from build123d import *

# Parameters (mm, degrees)
SKETCH1_R           = 23
BOSS_EXTRUDE1_DEPTH = 12
CUT_EXTRUDE1_DEPTH  = 13


with BuildPart() as part:
    # Sketch1 → Boss-Extrude1 (new body)
    with BuildSketch(Plane.XY):
        Circle(SKETCH1_R)
    extrude(amount=BOSS_EXTRUDE1_DEPTH)

    # Sketch2 → Cut-Extrude1 (cut, through all)
    with BuildSketch(Plane.XY.offset(12)):
        with BuildLine():
            Line((-1.669663439, 1.682), (1.669663439, 1.682))
            ThreePointArc((1.669663439, 1.682), (2.259858272, -0.714101248), (0.4, -2.336000856))
            Line((0.4, -2.336000856), (0.4, -5))
            Line((0.4, -5), (6.939400576, -5))
            add(Edge.make_bspline(
                [(-6.939400576, -5), (-6.939400576, -23.218031299), (0, -23.218031299), (6.939400576, -23.218031299), (6.939400576, -5)],
                knots=[1.570796327, 1.570796327, 1.570796327, 3.141592654, 3.141592654, 4.71238898, 4.71238898, 4.71238898], degree=2, weights=[1, 0.707106781, 1, 0.707106781, 1]))
            Line((-6.939400576, -5), (-0.4, -5))
            Line((-0.4, -5), (-0.4, -2.336000856))
            ThreePointArc((-0.4, -2.336000856), (-2.259858272, -0.714101248), (-1.669663439, 1.682))
        make_face()
        with BuildLine():
            Line((-6.939400576, 5), (6.939400576, 5))
            add(Edge.make_bspline(
                [(6.939400576, 5), (5.785687162, 25.074195607), (0, 25.074195607), (-5.785687162, 25.074195607), (-6.939400576, 5)],
                knots=[4.913142926, 4.913142926, 4.913142926, 6.283185307, 6.283185307, 7.653227688, 7.653227688, 7.653227688], degree=2, weights=[1, 0.77440564, 1, 0.77440564, 1]))
        make_face()
    extrude(amount=-CUT_EXTRUDE1_DEPTH, mode=Mode.SUBTRACT)


solid = part.part
Model file for the job. Use its own axes, mm. A direction names the side the tool comes from. Give positions to 0.01 mm unless a question says otherwise; leave off trailing zeros. Order: outer loops, then holes, each group sorted by start corner. A loop starts at its lowest first (then second) coordinate and runs counter-clockwise, first axis right, second up. Notation, with made-up numbers: M -36,-17 L -13,-17 A34 cw -13,17 Z; hole C -36.75,-12 d5. An arc over 180 degrees is marked long. Put each result on its own line as item: value. Start each with the question number.
(1) Tool access for faces 1 (the face through (22.96, -1.38, 5.92)), 2 (the face through (0, 1.682, 6)), 3 (the face through (0.4, -4, 6)): list every direction of +Z, -Z, +X, -X, +Y, -Y with a clear straight run to the whole face (end or side of a thin tool).
(2) Drill centre lines: L1, parallel to X at y = 0, z = 1.25; L2, parallel to X at y = -17.5, z = 7.75; L3, parallel to Y at x = 17, z = 0.5. Where is each one in solid material? Low to high. Write a range as [from, to].
(3) Pin check, flat tips, straight feed: pin 1 Ø1 at (x, z) = (-0.5, 6.5) entering from -Y; pin 2 Ø2 at (x, z) = (3.5, 5.5) entering from -Y; pin 3 Ø1 at (x, z) = (-11.5, 3) entering from +Y; pin 4 Ø6 at (x, z) = (2.5, 4.5) entering from +Y. Stop position of each tip, or through.
(4) Band-saw the part on D-D on x = -12.5. Give the cut face in (y, z).
(5) Band-saw the part on A-A on x = -6. Count the separate pieces of the cut face and the enclosed holes in it, then the cut area to 3 significant figures.
(6) Band-saw the part on B-B on x = 9. Give the cut face in (y, z).
(7) Pull direction Y, two halves, no side cores. Call faces 4 (the face through (-2.25, -0.75, 6.08)), 5 (the face through (-23, 0, 6)), 6 (the face through (5, 0, 12)), 7 (the face through (4, -5, 6)): released by +Y, released by -Y, zero draft, split by the parting line, or undercut.
Results below:
1. face 1: +Z, -Z, +X
1. face 2: +Z, -Z
1. face 3: +Z, -Z, -Y
2. L1: x = [-23, -2.37], [2.37, 23]
2. L2: x = [-14.92, -5.05], [5.05, 14.92]
2. L3: y = [-15.49, 15.49]
3. pin 1: stops at y = -5
3. pin 2: stops at y = -22.86
3. pin 3: stops at y = 20.2
3. pin 4: stops at y = 22.81
4. outline: M -19.31,0 L 19.31,0 L 19.31,12 L -19.31,12 Z
5. separate pieces: 3
5. enclosed holes: 0
5. area: 323 mm2
6. outline: M -21.17,0 L 21.17,0 L 21.17,12 L -21.17,12 Z
7. face 4: undercut
7. face 5: split by the parting line
7. face 6: zero draft
7. face 7: undercut
